Read the model definition and answer for the solid it produces. Units are mm, in the model's axes. Coordinates: 2 decimals unless noted, no trailing zeros. Order: outer loops, then holes, each group sorted by start corner. A loop starts at its lowest first (then second) coordinate and runs counter-clockwise, first axis right, second up. Notation, with made-up numbers: (77.25, 5) - (82.25, 5) arc R26 cw to (82.25, 31) - close; hole circle Ø10 at (68.5, 8.5). An arc over 180 degrees is marked (long way). Use one line per item in the form item = value.
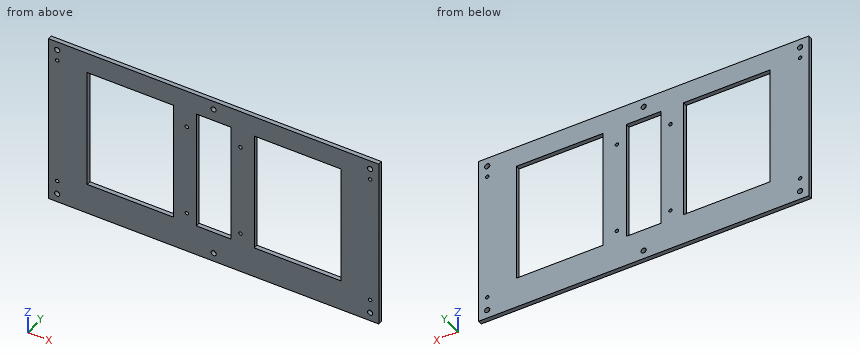
```python
from build123d import *

# Parameters (mm, degrees)
SKETCH1_W           = 382
SKETCH1_H           = 200
BOSS_EXTRUDE5_DEPTH = 5
SKETCH7_R           = 2
CUT_EXTRUDE4_DEPTH  = 5
SKETCH8_W           = 40
SKETCH8_H           = 140
SKETCH8_W_2         = 100
CUT_EXTRUDE5_DEPTH  = 10
SKETCH9_R           = 3
CUT_EXTRUDE6_DEPTH  = 10


with BuildPart() as part:
    # Sketch1 → Boss-Extrude5 (new body)
    with BuildSketch(Plane(origin=(0, 0, 0), x_dir=(1, 0, 0), z_dir=(0, 1, 0))):
        with Locations((0, 6)):
            Rectangle(SKETCH1_W, SKETCH1_H)
    extrude(amount=BOSS_EXTRUDE5_DEPTH)

    # Sketch7 → Cut-Extrude4 (cut)
    with BuildSketch(Plane(origin=(0, 5, 0), x_dir=(1, 0, 0), z_dir=(0, 1, 0))):
        with Locations((181, 80)):
            Circle(SKETCH7_R)
        with Locations((181, -70.8)):
            Circle(SKETCH7_R)
        with Locations((31, 58.6)):
            Circle(SKETCH7_R)
        with Locations((-31, 58.6)):
            Circle(SKETCH7_R)
        with Locations((-181, 80)):
            Circle(SKETCH7_R)
        with Locations((-181, -70.8)):
            Circle(SKETCH7_R)
        with Locations((31, -49.4)):
            Circle(SKETCH7_R)
        with Locations((-31, -49.4)):
            Circle(SKETCH7_R)
    extrude(amount=-CUT_EXTRUDE4_DEPTH, mode=Mode.SUBTRACT)

    # Sketch8 → Cut-Extrude5 (cut)
    with BuildSketch(Plane(origin=(0, 5, 0), x_dir=(1, 0, 0), z_dir=(0, 1, 0))):
        Rectangle(SKETCH8_W, SKETCH8_H)
        with Locations((97.15487949, 0)):
            Rectangle(SKETCH8_W_2, SKETCH8_H)
        with Locations((-96.318135121, 0)):
            Rectangle(SKETCH8_W_2, SKETCH8_H)
    extrude(amount=-CUT_EXTRUDE5_DEPTH, mode=Mode.SUBTRACT)

    # Sketch9 → Cut-Extrude6 (cut)
    with BuildSketch(Plane(origin=(0, 5, 0), x_dir=(1, 0, 0), z_dir=(0, 1, 0))):
        with Locations((181, 96)):
            Circle(SKETCH9_R)
        with Locations((181, -84)):
            Circle(SKETCH9_R)
        with Locations((-181, 96)):
            Circle(SKETCH9_R)
        with Locations((-181, -84)):
            Circle(SKETCH9_R)
        with Locations((0, 96)):
            Circle(SKETCH9_R)
        with Locations((0, -84)):
            Circle(SKETCH9_R)
    extrude(amount=-CUT_EXTRUDE6_DEPTH, mode=Mode.SUBTRACT)


solid = part.part
```
(1) Section C-C, the plane x = 117 is taken. Write down the section's boundary in (y, z).
Answer list:
outline = (0, -106) - (5, -106) - (5, -70) - (0, -70) - close; (0, 70) - (5, 70) - (5, 94) - (0, 94) - close
(2) Straight lines are drawn through the part: L1, parallel to X at y = 1.2, z = 84; L2, parallel to Z at x = 0, y = 1.4; L3, parallel to X at y = 4.15, z = -56.5. For each, find the intervals that lie inside material, in ascending order.
Answer list:
L1 = -191 to -184, -178 to -3, 3 to 178, 184 to 191
L2 = -106 to -99, -93 to -70, 70 to 81, 87 to 94
L3 = -191 to -146.32, -46.32 to -20, 20 to 47.15, 147.15 to 191
(3) Section B-B, the plane y = 3.55 is taken. State how many separate pieces and enclosed holes the cut face has, then the cut area to 3 significant figures.
Answer list:
separate_pieces = 1
enclosed_holes = 17
area = 42,500 mm2
(4) Section A-A, the plane z = 27 is taken. Write down the section's boundary in (x, y), then the cut area to 3 significant figures.
Answer list:
outline = (-191, 0) - (-146.32, 0) - (-146.32, 5) - (-191, 5) - close; (-46.32, 0) - (-20, 0) - (-20, 5) - (-46.32, 5) - close; (20, 0) - (47.15, 0) - (47.15, 5) - (20, 5) - close; (147.15, 0) - (191, 0) - (191, 5) - (147.15, 5) - close
area = 710 mm2
